Model file for the job. Use its own axes, mm. Round coordinates to 2 decimals unless told otherwise and drop trailing zeros. Order: outer loops, then holes, each group sorted by start corner. A loop starts at its lowest first (then second) coordinate and runs counter-clockwise, first axis right, second up. Notation, with made-up numbers: M -22.5,13.5 L 9.5,13.5 A26 cw 9.5,42.5 Z; hole C 74.5,86.5 d8. An arc over 180 degrees is marked long. Return JSON: item names as keys, results as strings. Group by question number.
Item 1: Pin check, flat tips, straight feed: pin 1 Ø1 at (x, y) = (10.5, 13.5) entering from +Z; pin 2 Ø8 at (x, y) = (28.5, 6) entering from -Z. Stop position of each tip, or through.
Item 2: Probe line 1 along Z through (x, y) = (31.5, 15); line 2 along Y through (x, z) = (2.5, 268.5); line 3 along X through (y, z) = (1.75, 138). List the from-to ranges inside material, lowest first.
Item 3: Slice it at A-A on y = 9. Write the cut outline in (x, z), then the cut area to 3 significant figures.
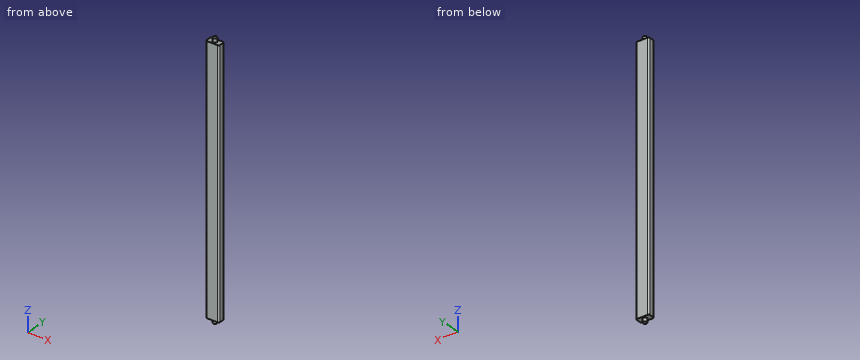
from build123d import *

# Parameters (mm, degrees)
F0_W          = 34
F0_H          = 18
F1_DEPTH      = 662
F2_R          = 5
F3_DEPTH      = 10
F3_DEPTH_BACK = 672
F4_R          = 3


with BuildPart() as f1:
    # F0 (on Top) → F1 (new body)
    with BuildSketch(Plane.XY):
        with Locations((17, 9)):
            Rectangle(F0_W, F0_H)
    extrude(amount=F1_DEPTH)

    # F2 (on face) → F3 (join, two sides)
    with BuildSketch(Plane(origin=(0, 0, 0), x_dir=(1, 0, 0), z_dir=(0, 0, -1))) as f3_sk:
        with Locations((17, -9)):
            Circle(F2_R)
    extrude(amount=F3_DEPTH)
    extrude(f3_sk.sketch, amount=-F3_DEPTH_BACK)

    # F4
    f4_edges = [f1.edges().sort_by_distance(p)[0] for p in [
        (0, 0, 331),
        (0, 18, 331),
        (34, 18, 331),
        (34, 0, 331),
    ]]
    fillet(f4_edges, radius=F4_R)


solid = f1.part
Output values:
{
 "1": {"pin 1": "z = 662", "pin 2": "z = 0"},
 "2": {"line 1": "0 to 662", "line 2": "0.04 to 17.96", "line 3": "0.27 to 33.73"},
 "3": {"outline": "M 0,0 L 12,0 L 12,-10 L 22,-10 L 22,0 L 34,0 L 34,662 L 22,662 L 22,672 L 12,672 L 12,662 L 0,662 Z", "area": "22,700 mm²"}
}
